CAD build for the part. Positions are in the model's coordinates, mm. A direction names the side the tool comes from. Give positions to 0.01 mm unless a question says otherwise; leave off trailing zeros. Write each loop counter-clockwise with the first axis right and the second up, starting at its lowest first coordinate (ties: lowest second). Pieces come first, ordered by that corner, then holes. Notation, with made-up numbers: (15, -29.75) - (53, -29.75) arc R32 ccw to (53, 9.25) - close; hole circle Ø1 at (75, 1). An arc over 180 degrees is marked (long way). Answer as a JSON object with one key per item and string values.
from build123d import *

# Parameters (mm, degrees)
SKETCH1_R           = 1.45
SKETCH1_RX          = 8.302080555
SKETCH1_RY          = 4.346497416
BOSS_EXTRUDE1_DEPTH = 5.85


with BuildPart() as part:
    # Sketch1 → Boss-Extrude1 (new body)
    with BuildSketch(Plane.XY):
        with BuildLine():
            Line((781.459168709, 464.852359197), (778.776092953, 464.852359197))
            Line((778.776092953, 464.852359197), (778.776092953, 461.952359197))
            Line((778.776092953, 461.952359197), (781.459168709, 461.952359197))
            Line((781.459168709, 461.952359197), (781.459168709, 455.852359197))
            Line((781.459168709, 455.852359197), (778.759168709, 455.852359197))
            Line((778.759168709, 455.852359197), (782.606547069, 438.402359197))
            ThreePointArc((782.606547069, 438.402359197), (787.659168709, 434.342389784), (792.711790348, 438.402359197))
            Line((792.711790348, 438.402359197), (796.559168709, 455.852359197))
            Line((796.559168709, 455.852359197), (793.859168709, 455.852359197))
            Line((793.859168709, 455.852359197), (793.859168709, 461.952359197))
            Line((793.859168709, 461.952359197), (796.542244464, 461.952359197))
            Line((796.542244464, 461.952359197), (796.542244464, 464.852359197))
            Line((796.542244464, 464.852359197), (793.859168709, 464.852359197))
            Line((793.859168709, 464.852359197), (793.859168709, 470.952359197))
            Line((793.859168709, 470.952359197), (796.559168709, 470.952359197))
            Line((796.559168709, 470.952359197), (792.711790348, 488.402359197))
            ThreePointArc((792.711790348, 488.402359197), (787.659168709, 492.46232861), (782.606547069, 488.402359197))
            Line((782.606547069, 488.402359197), (778.759168709, 470.952359197))
            Line((778.759168709, 470.952359197), (781.459168709, 470.952359197))
            Line((781.459168709, 470.952359197), (781.459168709, 464.852359197))
        make_face()
        with Locations((787.659168709, 488.402359197)):
            Circle(SKETCH1_R, mode=Mode.SUBTRACT)
        with Locations((787.659168709, 438.402359197)):
            Circle(SKETCH1_R, mode=Mode.SUBTRACT)
        with Locations((787.659168709, 463.402359197)):
            Circle(SKETCH1_R, mode=Mode.SUBTRACT)
        with Locations(Location((787.659168709, 475.448118238), (0, 0, 90))):
            Ellipse(SKETCH1_RX, SKETCH1_RY, mode=Mode.SUBTRACT)
        with Locations(Location((787.659168709, 451.356600156), (0, 0, -90))):
            Ellipse(SKETCH1_RX, SKETCH1_RY, mode=Mode.SUBTRACT)
    extrude(amount=BOSS_EXTRUDE1_DEPTH)


solid = part.part
(1) Flat gauge pins, fed straight in: P1, Ø2.5, axis at x = 787.66, y = 488.4, coming from the -Z side; P2, Ø1, axis at y = 450.5, z = 1, coming from the -X side; P3, Ø3, axis at y = 462, z = 1.5, coming from the -X side; P4, Ø3, axis at y = 468, z = 3.5, coming from the -X side. Where does each tip first touch, or does it go through?
Answer key:
{"P1": "passes through", "P2": "stops at x = 779.83", "P3": "stops at x = 778.78", "P4": "stops at x = 781.46"}
(2) Saw through at A-A, the plane x = 780.5. Give the cut face in (y, z), and give its area (3 significant figures).
Answer key:
{"outline": "(447.96, 0) - (455.85, 0) - (455.85, 5.85) - (447.96, 5.85) - close; (461.95, 0) - (464.85, 0) - (464.85, 5.85) - (461.95, 5.85) - close; (470.95, 0) - (478.85, 0) - (478.85, 5.85) - (470.95, 5.85) - close", "area": "109 mm²"}
(3) Saw through at C-C, the plane y = 466. Give the cut face in (x, z), and give its area (3 significant figures).
Answer key:
{"outline": "(781.46, 0) - (793.86, 0) - (793.86, 5.85) - (781.46, 5.85) - close", "area": "72.5 mm²"}
(4) Pull direction Y, two halves, no side cores. Call faces 1 (the face through (780, 455.852, 3)), 2 (the face through (790, 464, 5.85)), 3 (the face through (794.61, 447.01, 2.88)): pulls with the +Y half, pulls with the -Y half, needs draft (parallel to the pull), parting line crosses it, or undercut.
Answer key:
{"face 1": "undercut", "face 2": "needs draft", "face 3": "pulls with the -Y half"}
(5) Saw through at B-B, the plane z = 1.05. State how many separate pieces and enclosed holes the cut face has, and give its area (3 significant figures).
Answer key:
{"separate pieces": "1", "enclosed holes": "5", "area": "504 mm²"}
(6) 3-axis set-ups, long thin cutter, end or side, ignore diameter. For faces 4 (the face through (781.459, 459, 3)), 5 (the face through (787.76, 492.46, 2.88)), 6 (the face through (793.859, 459, 3)): which of +Z, -Z, +X, -X, +Y, -Y reach the whole face in a straight line?
Answer key:
{"face 4": "+Z, -Z, -X", "face 5": "+Z, -Z, +Y", "face 6": "+Z, -Z, +X"}
(7) Probe L1, parallel to Y at x = 788.25, z = 0.9; L2, parallel to Y at x = 785.5, z = 2.05; L3, parallel to Y at x = 789.75, z = 3.2. List the from-to ranges inside material, lowest first. Write a range as [from, to].
Answer key:
{"L1": "y = [434.38, 437.08], [439.73, 443.13], [459.58, 462.08], [464.73, 467.22], [483.67, 487.08], [489.73, 492.43]", "L2": "y = [434.81, 444.15], [458.56, 468.24], [482.65, 491.99]", "L3": "y = [434.78, 444.08], [458.64, 468.17], [482.73, 492.02]"}
